Model file for the job. Use its own axes, mm. Face numbers are marked on the shaded views. A direction names the side the tool comes from. Coordinates: 2 decimals unless noted, no trailing zeros. Loops run counter-clockwise (first coordinate to the right, second up) from the corner with the lowest first, then second, coordinate; pieces in that order, holes last. Notation, with made-up numbers: (5, -8.5) - (45, -8.5) arc R7 cw to (45, 4.5) - close; hole circle Ø8 at (76.25, 20). An arc over 180 degrees is marked (long way). Write each question's results on one line, items separated by ' | '. Start each with the question number.
```python
from build123d import *

# Parameters (mm, degrees)
SKETCH1_R           = 1.651
BOSS_EXTRUDE1_DEPTH = 10.414
SKETCH2_W           = 12.7
SKETCH2_H           = 4.1148
SKETCH2_H_2         = 4.0767
CUT_EXTRUDE1_DEPTH  = 7.35


with BuildPart() as part:
    # Sketch1 → Boss-Extrude1 (new body)
    with BuildSketch(Plane.XY):
        with BuildLine():
            Line((-71.178896696, 3.175), (-50.858896696, 3.175))
            ThreePointArc((-50.858896696, 3.175), (-47.683896696, 0), (-50.858896696, -3.175))
            Line((-50.858896696, -3.175), (-71.178896696, -3.175))
            ThreePointArc((-71.178896696, -3.175), (-74.353896696, 0), (-71.178896696, 3.175))
        make_face()
        with Locations((-50.858896696, 0)):
            Circle(SKETCH1_R, mode=Mode.SUBTRACT)
        with Locations((-71.178896696, 0)):
            Circle(SKETCH1_R, mode=Mode.SUBTRACT)
    extrude(amount=BOSS_EXTRUDE1_DEPTH)

    # Sketch2 → Cut-Extrude1 (cut, through all)
    with BuildSketch(Plane(origin=(0, 3.175, 0), x_dir=(1, 0, 0), z_dir=(0, 1, 0))):
        with Locations((-68.003896696, -5.207)):
            Rectangle(SKETCH2_W, SKETCH2_H)
        with Locations((-48.953896696, -5.207)):
            Rectangle(SKETCH2_W, SKETCH2_H_2)
    extrude(amount=-CUT_EXTRUDE1_DEPTH, mode=Mode.SUBTRACT)


solid = part.part
```
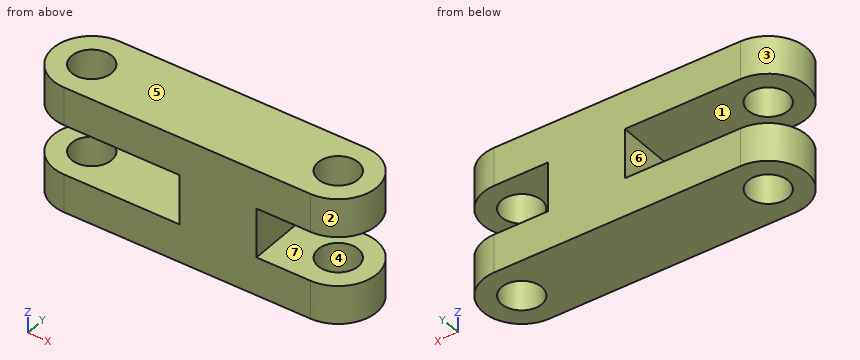
Q1. Which spindle directions (+Z, -Z, +X, -X, +Y, -Y) get a long thin tool onto all of the face, cutting with end or side? Do the marked faces 5, 6 and 7. Say none if no direction does.
Q2. Cut at C-C (z = 9.5). List the corners of the cut face in (x, y) (3 decimals).
Q3. Cut at A-A (x = -64). List the corners of the cut face in (y, z) (3 decimals).
Q4. Mould opens along X. For the marked faces 1, 2, 3 and 4 say: +X half, -X half, draft (parallel to the pull), parting line (faces both ways), or undercut.
Q5. Drill centre lines: L1, parallel to X at y = 0, z = 0.9; L2, parallel to Z at x = -66, y = -2.5; L3, parallel to Y at x = -72.5, z = 9.5. Where is each one in solid material? Low to high. Write a range as from..to.
Q6. Cut at D-D (x = -70). List the corners of the cut face in (y, z) (3 decimals), and give its area (3 significant figures).
Q7. Cut at B-B (y = -1). List the corners of the cut face in (x, z).
Q8. Pin check, flat tips, straight feed: pin 1 (1.2 mm diameter, centred on y = -0.5, z = 6, fed in from -X); pin 2 (2 mm diameter, centred on y = -1.5, z = 3, fed in from -X); pin 3 (2 mm diameter, centred on y = 1, z = 6, fed in from +X). Stop position of each tip, or through.
Check result:
1) face 5: +Z, +X, -X, +Y, -Y | face 6: -X, +Y, -Y | face 7: +X, +Y, -Y
2) outline: (-71.179, -3.175) - (-50.859, -3.175) arc R3.175 ccw to (-50.859, 3.175) - (-71.179, 3.175) arc R3.175 ccw to start; hole circle Ø3.302 at (-71.179, 0); hole circle Ø3.302 at (-50.859, 0)
3) outline: (-3.175, 0) - (3.175, 0) - (3.175, 3.15) - (-3.175, 3.15) - close; (-3.175, 7.264) - (3.175, 7.264) - (3.175, 10.414) - (-3.175, 10.414) - close
4) face 1: draft | face 2: +X half | face 3: -X half | face 4: undercut
5) L1: -74.35..-72.83, -69.53..-52.51, -49.21..-47.68 | L2: 0..3.15, 7.26..10.41 | L3: -2.89..-0.99, 0.99..2.89
6) outline: (-3.175, 0) - (-1.156, 0) - (-1.156, 3.15) - (-3.175, 3.15) - close; (-3.175, 7.264) - (-1.156, 7.264) - (-1.156, 10.414) - (-3.175, 10.414) - close; (1.156, 0) - (3.175, 0) - (3.175, 3.15) - (1.156, 3.15) - close; (1.156, 7.264) - (3.175, 7.264) - (3.175, 10.414) - (1.156, 10.414) - close | area: 25.4 mm²
7) outline: (-74.19, 0) - (-72.49, 0) - (-72.49, 3.15) - (-74.19, 3.15) - close; (-74.19, 7.26) - (-72.49, 7.26) - (-72.49, 10.41) - (-74.19, 10.41) - close; (-69.87, 0) - (-52.17, 0) - (-52.17, 3.17) - (-55.3, 3.17) - (-55.3, 7.25) - (-52.17, 7.25) - (-52.17, 10.41) - (-69.87, 10.41) - (-69.87, 7.26) - (-61.65, 7.26) - (-61.65, 3.15) - (-69.87, 3.15) - close; (-49.55, 0) - (-47.85, 0) - (-47.85, 3.17) - (-49.55, 3.17) - close; (-49.55, 7.25) - (-47.85, 7.25) - (-47.85, 10.41) - (-49.55, 10.41) - close
8) pin 1: x = -61.65 | pin 2: x = -74.31 | pin 3: x = -55.3
